```python
from build123d import *

# Parameters (mm, degrees)
PAD_DEPTH       = 4
POCKET_DEPTH    = 2
POCKET001_DEPTH = 5


with BuildPart() as part:
    # Sketch001 → Pad (new body)
    with BuildSketch(Plane.YZ):
        Polygon((56.5, 56), (56.5, 39), (56.5, 7.155514), (51.4, 10.1), (51.4, -10.1), (56.5, -7.155514), (56.5, -40), (56.5, -57), (39.5, -57), (7.113249, -57), (10, -62), (-10, -62), (-7.113249, -57), (-39.5, -57), (-56.5, -57), (-56.5, -40), (-56.5, -7.113249), (-61.5, -10), (-61.5, 10), (-56.5, 7.113249), (-56.5, 39), (-56.5, 56), (-39.5, 56), (-7.155514, 56), (-10.1, 50.9), (10.1, 50.9), (7.155514, 56), (39.5, 56), align=None)
    extrude(amount=PAD_DEPTH)

    # Sketch → Pocket (cut)
    with BuildSketch(Plane.YZ.offset(4)):
        Polygon((-40, 40), (-18.6, 40), (-18.6, 62), (18.6, 62), (18.6, 40), (40, 40), (40, 18.6), (62, 18.6), (62, -18.6), (40, -18.6), (40, -40), (18.6, -40), (18.6, -62), (-18.6, -62), (-18.6, -40), (-40, -40), (-40, -18.6), (-62, -18.6), (-62, 18.6), (-40, 18.6), align=None)
    extrude(amount=-POCKET_DEPTH, mode=Mode.SUBTRACT)

    # Sketch002 → Pocket001 (cut)
    with BuildSketch(Plane.YZ.offset(4)):
        Polygon((-44, 43.5), (-44, 22.6), (-56.5, 22.6), (-56.5, 56), (-23.1, 56), (-23.1, 43.5), align=None)
        Polygon((23.1, 43.5), (23.1, 56), (56.5, 56), (56.5, 22.6), (44, 22.6), (44, 43.5), align=None)
        Polygon((-56.5, -23.6), (-44, -23.6), (-44, -44.5), (-23.1, -44.5), (-23.1, -57), (-56.5, -57), align=None)
        Polygon((23.1, -44.5), (44, -44.5), (44, -23.6), (56.5, -23.6), (56.5, -57), (23.1, -57), align=None)
    extrude(amount=-POCKET001_DEPTH, mode=Mode.SUBTRACT)


solid = part.part
```
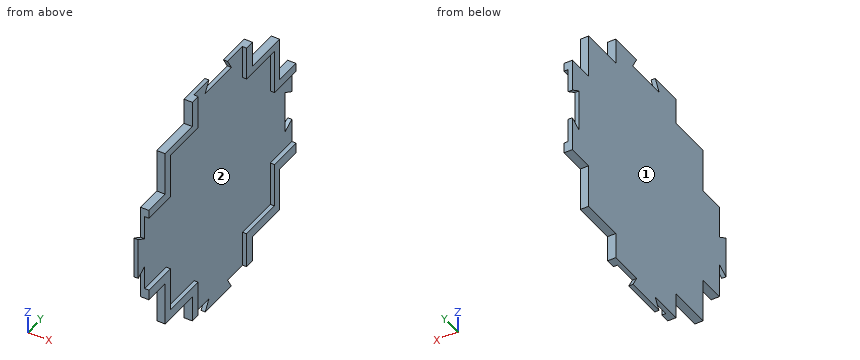
For this review, take the finished solid that the model builds, in its own axes (mm). Face numbers are marked on the shaded views. Give positions to 0.01 mm unless a question says otherwise; leave off trailing zeros. Order: outer loops, then holes, each group sorted by start corner. A loop starts at its lowest first (then second) coordinate and runs counter-clockwise, first axis right, second up.
1) Take a section at D-D (y = -5). Give the boundary of the cut face in (x, z), then the cut area to 3 significant figures.
2) Take a section at B-B (z = 47.5). Give the boundary of the cut face in (x, y), then the cut area to 3 significant figures.
3) Take a section at C-C (x = 3.3). State how many separate pieces and enclosed holes the cut face has, then the cut area to 3 significant figures.
4) Take a section at A-A (y = -42). Give the boundary of the cut face in (x, z).
5) Insertion check: pin 1 (0.6 mm diameter, centred on x = 2.5, y = -48, fed in from -Z); pin 2 (1.5 mm diameter, centred on x = 3, z = 39, fed in from -Y); pin 3 (0.6 mm diameter, centred on x = 0.5, y = 2.5, fed in from +Z); pin 4 (1.5 mm diameter, centred on x = 3, y = 14.5, fed in from +Z). Each pin has a flat end and moves straight along its axis. Give the tip position at first contact, or say it passes through.
6) Wall thickness on line 1 (Z direction, x = 2.45, y = -45); line 2 (Y direction, x = 3.6, z = -45.5); line 3 (Z direction, x = 3.5, y = -43.5): over which ranges is each line inside the solid? List them lowest first.
7) The part is to be moulded in two halves that separate along Y. For the marked faces 1 and 2, say which applies: released by +Y, released by -Y, zero draft, split by the parting line, or undercut.
Derived:
1. outline: (0, -62) - (2, -62) - (2, 50.9) - (0, 50.9) - close
1. area: 226 mm2
2. outline: (0, -23.1) - (4, -23.1) - (4, -18.6) - (2, -18.6) - (2, 18.6) - (4, 18.6) - (4, 23.1) - (0, 23.1) - close
2. area: 110 mm2
3. separate pieces: 4
3. enclosed holes: 0
3. area: 1,200 mm2
4. outline: (0, -44.5) - (4, -44.5) - (4, -18.6) - (2, -18.6) - (2, 18.6) - (4, 18.6) - (4, 43.5) - (0, 43.5) - close
5. pin 1: stops at z = -23.6
5. pin 2: stops at y = -44
5. pin 3: stops at z = 50.9
5. pin 4: passes through
6. line 1: z = -23.6 to -18.6, 18.6 to 22.6
6. line 2: y = -23.1 to -18.6, 18.6 to 23.1
6. line 3: z = -44.5 to -18.6, 18.6 to 43.5
7. face 1: zero draft
7. face 2: undercut
